Check sheet for the drawn part. Datum: minimum x, y, z corner. Units: mm. Round coordinates to 2 decimals unless told otherwise and drop trailing zeros. Loops run counter-clockwise (first coordinate to the right, second up) from the corner with the lowest first, then second, coordinate; pieces in that order, holes last. Notation, with made-up numbers: (24, 12) -> (40, 12) arc R11 cw to (40, 18) -> close; hole circle Ø8 at (28.5, 33.5). An arc over 180 degrees is marked (long way). Return JSON: item names as keys, results as strings.
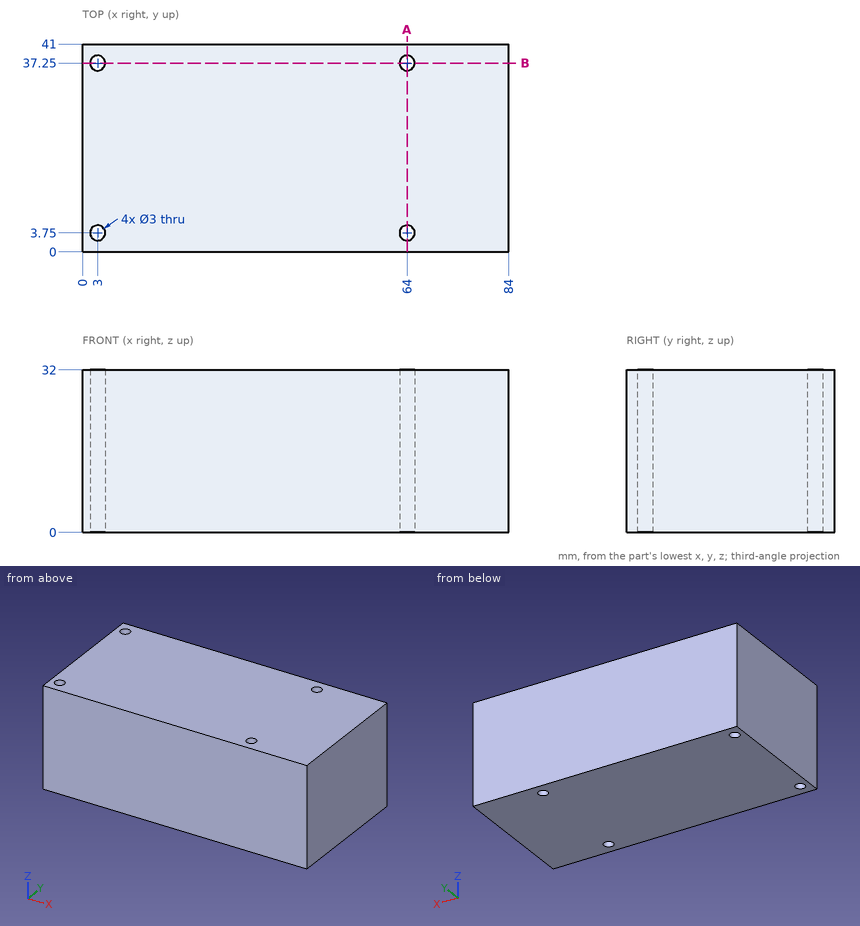
Q1. Section check B-B (y = 37.25). Record the boundary of the cut face in (x, z).
Results list:
{"outline": "(0, 0) -> (1.5, 0) -> (1.5, 32) -> (0, 32) -> close; (4.5, 0) -> (62.5, 0) -> (62.5, 32) -> (4.5, 32) -> close; (65.5, 0) -> (84, 0) -> (84, 32) -> (65.5, 32) -> close"}
Q2. Section check A-A (x = 64). Record the boundary of the cut face in (y, z), then the cut area to 3 significant figures.
Results list:
{"outline": "(0, 0) -> (2.25, 0) -> (2.25, 32) -> (0, 32) -> close; (5.25, 0) -> (35.75, 0) -> (35.75, 32) -> (5.25, 32) -> close; (38.75, 0) -> (41, 0) -> (41, 32) -> (38.75, 32) -> close", "area": "1,120 mm^2"}
Q3. Material ranges on line 1 (Y direction, x = 64, z = 18.5); line 2 (X direction, y = 37.25, z = 12); line 3 (X direction, y = 3, z = 19), recorded low to high.
Results list:
{"line 1": "0 to 2.25, 5.25 to 35.75, 38.75 to 41", "line 2": "0 to 1.5, 4.5 to 62.5, 65.5 to 84", "line 3": "0 to 1.7, 4.3 to 62.7, 65.3 to 84"}
